Part model, mm, in its own coordinate system. A direction names the side the tool comes from. Coordinates: 2 decimals unless noted, no trailing zeros. Write each loop counter-clockwise with the first axis right and the second up, starting at its lowest first coordinate (ties: lowest second). Pieces come first, ordered by that corner, then holes. Notation, with made-up numbers: M -36,25 L -29,25 A13 ccw -29,43 Z; hole C 43.5,23.25 d6. An arc over 180 degrees is marked long. Use a Markdown table: item, result. Add a question column.
Q1. Pin check, flat tips, straight feed: pin 1 Ø4 at (y, z) = (-16.5, 57.5) entering from +X; pin 2 Ø2 at (x, y) = (11.5, -27) entering from -Z; pin 3 Ø18 at (x, z) = (-2, 39) entering from +Y; pin 4 Ø8 at (x, y) = (6, -12) entering from +Z. Stop position of each tip, or through.
Q2. Tool access for faces 5 (the flat face through (-4, 0, 400)), 6 (the flat face through (-6, -20, 66)): list every direction of +Z, -Z, +X, -X, +Y, -Y with a clear straight run to the whole face (end or side of a thin tool).
Q3. Slice it at A-A on y = -5.5. Write the cut outline in (x, z), then the cut area to 3 significant figures.
Q4. Slice it at D-D on z = 279. Write the cut outline in (x, y).
Q5. Slice it at C-C on z = 87.5. Write the cut outline in (x, y) (3 decimals), then the cut area to 3 significant figures.
Q6. Slice it at B-B on z = 0. Write the cut outline in (x, y) (3 decimals).
Q7. Wall check: L1, parallel to Y at x = -4.5, z = 60.5 (3 decimals); L2, parallel to X at y = -18, z = 195; L3, parallel to Y at x = -30.5, z = 334. Give the ranges that are in metal, low to high. Write a range as from..to.
Q8. Mould opens along X. For faces 1 (the cylindrical face through (1.302, -9.86, 499.915)), 2 (the cylindrical face through (2.17, -26.22, -9.76)), 3 (the flat face through (-5, -20, 398)), 4 (the cylindrical face through (1.75, -9.86, 514.94)) say: released by +X, released by -X, zero draft, split by the parting line, or undercut.
Autodesk Inventor part; units mm, degrees
ref_plane "YZ Plane" through (0, 0, 0) normal (1, 0, 0) x (0, 1, 0)
ref_plane "XZ Plane" through (0, 0, 0) normal (0, 1, 0) x (-1, 0, 0)
ref_plane "XY Plane" through (0, 0, 0) normal (0, 0, 1) x (1, 0, 0)
sketch "Sketch2" plane through (0, 0, 0) normal (0, 1, 0) x (-1, 0, 0)
  circle A0 centre (0, 490) radius 10
  circle A1 centre (0, 0) radius 10
  line L0 (24.5876, 494.5222) -> (49.3695, 359.7814)
  line L1 (50.7256, 334.0357) -> (21.9944, -40.0968)
  line L2 (18.9282, -41.6321) -> (-24.072, -14.3293)
  line L3 (-25, -12.6409) -> (-25, 490)
  arc A2 (24.5876, 494.5222) -> (-25, 490) centre (0, 490) ccw
  line L4 (0, -154.4311) -> (0, 629.0893) construction
  arc A3 (18.9282, -41.6321) -> (21.9944, -40.0968) centre (20.0003, -39.9437) ccw
  arc A4 (-25, -12.6409) -> (-24.072, -14.3293) centre (-23, -12.6409) ccw
  arc A5 (50.7256, 334.0357) -> (49.3695, 359.7814) centre (-48.9808, 341.6925) ccw
  line L5 (-17, 19.4683) -> (-17, 467.2676)
  line L6 (43.2667, 341.388) -> (18.4452, 18.1672)
  line L7 (15.4511, 16.5882) -> (5, 22.6222)
  line L8 (4, 24.3542) -> (4, 456.3028)
  line L9 (4.5133, 457.6406) -> (17.3407, 471.896)
  line L10 (-13.6891, 468.7781) -> (-4.6891, 460.9668)
  line L11 (-4, 459.4563) -> (-4, 27.5077)
  line L12 (-4.6676, 26.0162) -> (-13.6676, 17.9767)
  line L13 (-69.1212, 0) -> (71.8613, 0) construction
  line L14 (20.7944, 470.92) -> (42.7242, 351.6863)
  arc A6 (43.2667, 341.388) -> (42.7242, 351.6863) centre (3.3841, 344.4507) ccw
  arc A7 (-17, 19.4683) -> (-13.6676, 17.9767) centre (-15, 19.4683) ccw
  arc A8 (-4.6676, 26.0162) -> (-4, 27.5077) centre (-6, 27.5077) ccw
  arc A9 (4, 24.3542) -> (5, 22.6222) centre (6, 24.3542) ccw
  arc A10 (15.4511, 16.5882) -> (18.4452, 18.1672) centre (16.4511, 18.3203) ccw
  arc A11 (4.5133, 457.6406) -> (4, 456.3028) centre (6, 456.3028) ccw
  arc A12 (20.7944, 470.92) -> (17.3407, 471.896) centre (18.8274, 470.5582) ccw
  arc A13 (-13.6891, 468.7781) -> (-17, 467.2676) centre (-15, 467.2676) ccw
  arc A14 (-4, 459.4563) -> (-4.6891, 460.9668) centre (-6, 459.4563) ccw
  circle A15 centre (24.5876, 339.2417) radius 4
  circle A16 centre (-9.1676, 339.2417) radius 4
  point P0 (51.7209, 346.9967)
  point P1 (-17, 15)
  point P2 (18.202, 15)
  dimension "d0" = 20
  dimension "d1" = 20
  dimension "d2" = 490
  dimension "d3" = 15
  dimension "d4" = 10.421
  dimension "d6" = 25
  dimension "d7" = 25
  dimension "d8" = 25
  dimension "d9" = 150
  dimension "d10" = 2
  dimension "d11" = 100
  dimension "d14" = 15
  dimension "d15" = 15
  dimension "d16" = 8
  dimension "d18" = 8
  dimension "d19" = 8
  dimension "d20" = 60
  dimension "d21" = 40
  dimension "d22" = 8
  dimension "d23" = 25
  dimension "d24" = 25
  dimension "d25" = 2
  dimension "d28" = 8
extrude "Extrusion1" add sketch "Sketch2" against normal blind 32.625 contours L0 A5 L1 A3 L2 A4 L3 A2 | L5 A13 L10 A14 L11 A8 L12 A7 | L6 A10 L7 A9 L8 A11 L9 A12 L14 A6
extrude "Extrusion2" [suppressed]
sketch "Sketch3" plane through (0, 0, 0) normal (1, 0, 0) x (0, 1, 0)
  line L0 (0, -41.6321) -> (-32.625, -41.6321) construction
  line L1 (-32.625, 515) -> (-32.625, 490) construction
  line L2 (0, 490) -> (0, 515) construction
  line L3 (0, 515) -> (0, 325)
  line L4 (0, 325) -> (-20, 132.3117)
  line L5 (-20, 132.3117) -> (-20, -41.6321)
  line L6 (-20, -41.6321) -> (-40, -41.6321)
  line L7 (-40, -41.6321) -> (-40, 132.3117)
  line L8 (-40, 132.3117) -> (-20, 325)
  line L9 (-20, 325) -> (-20, 515)
  line L10 (-20, 515) -> (0, 515)
  point P0 (0, 0)
  point P1 (-32.625, 494.5222)
  point P2 (0, 494.5222)
  dimension "d11" = 100
  dimension "d29" = 20
  dimension "d30" = 190
  dimension "d31" = 20
extrude "Extrusion3" cut sketch "Sketch3" along normal through all both and the other way through all keep common part
equation "\"d1\" = d0"
equation "\"d6\" = 0.5 * d1 + d3"
equation "\"d7\" = d6"
equation "\"d8\" = d6"
equation "\"d18\" = d16"
equation "\"d19\" = d16"
equation "\"d22\" = d16"
equation "\"d23\" = 0.5 * d0 + d3"
equation "\"d24\" = d23"
properties part number "Profile_Straight" material "Aluminum 6061"
Recorded:
| question | item | result |
|---|---|---|
| 1 | pin 1 | through |
| 1 | pin 2 | z = -22.95 |
| 1 | pin 3 | y = -20 |
| 1 | pin 4 | z = 514.92 |
| 2 | face 5 | +Z, -Z, +X, -X, +Y |
| 2 | face 6 | -Z, +X, -X, +Y |
| 3 | outline | M -50.73,334.04 L -45.96,272.01 L 25,272.01 L 25,490 A25 ccw -24.59,494.52 L -49.37,359.78 A100 ccw Z; hole C -24.59,339.24 d8; hole C 0,490 d20; hole C 9.17,339.24 d8 |
| 3 | area | 15,200 mm² |
| 4 | outline | M -46.5,-24.77 L 25,-24.77 L 25,-4.77 L -46.5,-4.77 Z |
| 5 | outline | M -31.793,-32.625 L 25,-32.625 L 25,-20 L -31.793,-20 Z |
| 5 | area | 717 mm² |
| 6 | outline | M -25.074,-32.625 L -10,-32.625 L -10,-20 L -25.074,-20 Z; M 10,-32.625 L 25,-32.625 L 25,-20 L 10,-20 Z |
| 7 | L1 | -32.625..-20 |
| 7 | L2 | -40.05..25 |
| 7 | L3 | -20..0 |
| 8 | face 1 | undercut |
| 8 | face 2 | undercut |
| 8 | face 3 | zero draft |
| 8 | face 4 | split by the parting line |
